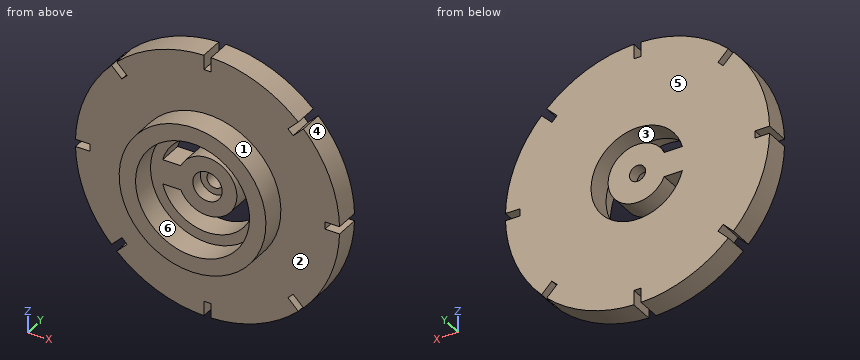
```python
from build123d import *

# Parameters (mm, degrees)
BOSS_EXTRUDE1_DEPTH = 5
SKETCH2_R           = 27
BOSS_EXTRUDE2_DEPTH = 5
SKETCH4_R           = 3
CUT_EXTRUDE1_DEPTH  = 2.5
CUT_EXTRUDE2_DEPTH  = 39.509739028
SKETCH6_W           = 4.309180809
SKETCH6_H           = 1.5
CUT_EXTRUDE3_DEPTH  = 40.471508712
CIRPATTERN1_COUNT   = 8
SKETCH7_R           = 1.65
CUT_EXTRUDE4_DEPTH  = 40.457255353


with BuildPart() as part:
    # Sketch1 → Boss-Extrude1 (new body)
    with BuildSketch(Plane(origin=(0, 0, 0), x_dir=(1, 0, 0), z_dir=(0, 1, 0))):
        with BuildLine():
            ThreePointArc((0, -15), (15, 0), (0, 15))
            ThreePointArc((0, 15), (-15, 0), (0, -15))
        make_face()
        with BuildLine():
            ThreePointArc((0, -11.65), (11.65, 0), (0, 11.65))
            ThreePointArc((0, 11.65), (-11.65, 0), (0, -11.65))
        make_face(mode=Mode.SUBTRACT)
    extrude(amount=BOSS_EXTRUDE1_DEPTH)

    # Sketch2 → Boss-Extrude2 (add)
    with BuildSketch(Plane(origin=(0, 5, 0), x_dir=(1, 0, 0), z_dir=(0, 1, 0))):
        with Locations(Location((0, 0, 0), (0, 0, 270))):
            Circle(SKETCH2_R)
    extrude(amount=BOSS_EXTRUDE2_DEPTH)

    # Sketch4 → Cut-Extrude1 (cut)
    with BuildSketch(Plane.XZ.offset(-5)):
        with Locations(Location((0, 0, 0), (0, 0, 270))):
            Circle(SKETCH4_R)
    extrude(amount=-CUT_EXTRUDE1_DEPTH, mode=Mode.SUBTRACT)

    # Sketch5 → Cut-Extrude2 (cut, through all)
    with BuildSketch(Plane.XZ.offset(-5)):
        with BuildLine():
            Line((-9.16515139, 2.5), (-5.454356057, 2.5))
            ThreePointArc((-5.454356057, 2.5), (6, 0), (-5.454356057, -2.5))
            Line((-5.454356057, -2.5), (-9.16515139, -2.5))
            ThreePointArc((-9.16515139, -2.5), (9.5, 0), (-9.16515139, 2.5))
        make_face()
    extrude(amount=-CUT_EXTRUDE2_DEPTH, mode=Mode.SUBTRACT)

    # Sketch6 → Cut-Extrude3 (cut, through all)
    with BuildSketch(Plane(origin=(0, 10, 0), x_dir=(1, 0, 0), z_dir=(0, 1, 0))):
        with Locations((-26.154590404, 0)):
            Rectangle(SKETCH6_W, SKETCH6_H)
    cut_extrude3 = extrude(amount=-CUT_EXTRUDE3_DEPTH, mode=Mode.SUBTRACT)

    # CirPattern1: Cut-Extrude3 ×8 about axis
    cirpattern1_axis = Axis((0, 0, 0), (0, 1, 0))
    for i in range(1, CIRPATTERN1_COUNT):
        add(cut_extrude3.rotate(cirpattern1_axis, i * 360 / CIRPATTERN1_COUNT), mode=Mode.SUBTRACT)

    # Sketch7 → Cut-Extrude4 (cut, through all)
    with BuildSketch(Plane(origin=(0, 10, 0), x_dir=(1, 0, 0), z_dir=(0, 1, 0))):
        with Locations(Location((0, 0, 0), (0, 0, 270))):
            Circle(SKETCH7_R)
    extrude(amount=-CUT_EXTRUDE4_DEPTH, mode=Mode.SUBTRACT)


solid = part.part
```
The model under review builds one solid part; all positions refer to its coordinate system, in mm. Face numbers are marked on the shaded views. A direction names the side the tool comes from. Round coordinates to 2 decimals unless told otherwise and drop trailing zeros. Loops run counter-clockwise (first coordinate to the right, second up) from the corner with the lowest first, then second, coordinate; pieces in that order, holes last. Notation, with made-up numbers: (17.5, 69) -> (65.5, 69) arc R7 ccw to (65.5, 76) -> close; hole circle Ø1 at (-24.5, -33). An arc over 180 degrees is marked (long way). Answer in a Markdown table with one row per item.
1) Tool access review of the marked faces 5 and 6: name each direction out of +Z, -Z, +X, -X, +Y, -Y from which nothing blocks a thin tool from reaching the whole face with its end or side.
Taken from the geometry:
| item | result |
|---|---|
| face 5 | +Z, -Z, +X, -X, +Y |
| face 6 | -Y |
2) Consider section D-D, the plane y = 1.25. Write out the cut boundary in (x, z), plus the area to 3 significant figures.
Taken from the geometry:
| item | result |
|---|---|
| outline | circle Ø30 at (0, 0); hole circle Ø23.3 at (0, 0) |
| area | 280 mm² |
3) Consider section C-C, the plane z = 7. Write out the cut boundary in (x, y), plus the area to 3 significant figures.
Taken from the geometry:
| item | result |
|---|---|
| outline | (-26.08, 5) -> (-13.27, 5) -> (-13.27, 0) -> (-9.31, 0) -> (-9.31, 5) -> (-6.42, 5) -> (-6.42, 10) -> (-26.08, 10) -> close; (6.42, 5) -> (9.31, 5) -> (9.31, 0) -> (13.27, 0) -> (13.27, 5) -> (26.08, 5) -> (26.08, 10) -> (6.42, 10) -> close |
| area | 236 mm² |
4) Consider section A-A, the plane x = 0. Write out the cut boundary in (y, z).
Taken from the geometry:
| item | result |
|---|---|
| outline | (0, -15) -> (5, -15) -> (5, -24) -> (10, -24) -> (10, -9.5) -> (5, -9.5) -> (5, -11.65) -> (0, -11.65) -> close; (0, 11.65) -> (5, 11.65) -> (5, 9.5) -> (10, 9.5) -> (10, 24) -> (5, 24) -> (5, 15) -> (0, 15) -> close; (5, -6) -> (10, -6) -> (10, -1.65) -> (7.5, -1.65) -> (7.5, -3) -> (5, -3) -> close; (5, 3) -> (7.5, 3) -> (7.5, 1.65) -> (10, 1.65) -> (10, 6) -> (5, 6) -> close |
5) For pin 1 Ø0.9 at (x, y) = (-25.5, 7.5) entering from -Z; pin 2 Ø1 at (y, z) = (7, -10.5) entering from +X; pin 3 Ø1.9 at (x, y) = (-7, 6.5) entering from -Z; pin 4 Ø5 at (x, z) = (0, 0) entering from +Y, all flat-tipped, find the tip position at first contact; note any pin that passes through.
Taken from the geometry:
| item | result |
|---|---|
| pin 1 | stops at z = -10.07 |
| pin 2 | stops at x = 25.08 |
| pin 3 | stops at z = -26.31 |
| pin 4 | stops at y = 10 |
6) Wall thickness on line 1 along X through (y, z) = (6.8, 0); line 2 along X through (y, z) = (7.55, 0); line 3 along Z through (x, y) = (4, 5.75): over which ranges is each line inside the solid? List them lowest first.
Taken from the geometry:
| item | result |
|---|---|
| line 1 | x = -24 to -3, 3 to 6, 9.5 to 24 |
| line 2 | x = -24 to -1.65, 1.65 to 6, 9.5 to 24 |
| line 3 | z = -26.7 to -8.62, -4.47 to 4.47, 8.62 to 26.7 |
7) Consider section B-B, the plane z = 0. Write out the cut boundary in (x, y).
Taken from the geometry:
| item | result |
|---|---|
| outline | (-24, 5) -> (-15, 5) -> (-15, 0) -> (-11.65, 0) -> (-11.65, 5) -> (-3, 5) -> (-3, 7.5) -> (-1.65, 7.5) -> (-1.65, 10) -> (-24, 10) -> close; (1.65, 7.5) -> (3, 7.5) -> (3, 5) -> (6, 5) -> (6, 10) -> (1.65, 10) -> close; (9.5, 5) -> (11.65, 5) -> (11.65, 0) -> (15, 0) -> (15, 5) -> (24, 5) -> (24, 10) -> (9.5, 10) -> close |
8) Draft analysis for pull direction X (two halves, no side actions). For the marked faces 1, 2, 3 and 4, state which applies: pulls with the +X half, pulls with the -X half, needs draft (parallel to the pull), parting line crosses it, or undercut.
Taken from the geometry:
| item | result |
|---|---|
| face 1 | parting line crosses it |
| face 2 | needs draft |
| face 3 | undercut |
| face 4 | pulls with the +X half |
